Geometry check sheet. Reference: the model listing, model coordinates, mm. Face numbers are marked on the shaded views. Give positions to 0.01 mm unless a question says otherwise; leave off trailing zeros. Order: outer loops, then holes, each group sorted by start corner. A loop starts at its lowest first (then second) coordinate and runs counter-clockwise, first axis right, second up.
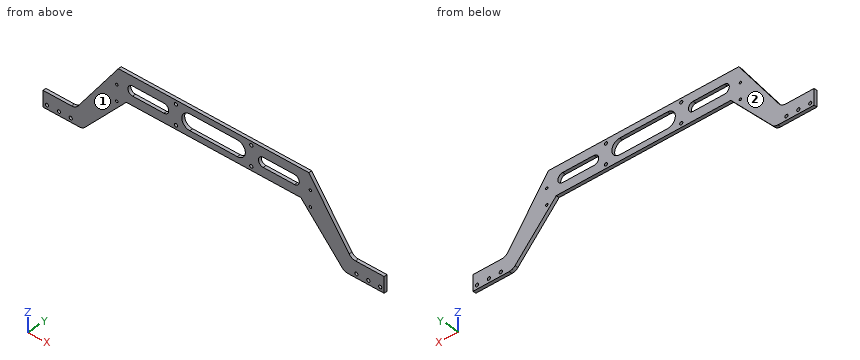
from build123d import *

# Parameters (mm, degrees)
SKETCH_2_R          = 2
EXTRUDE_1_DEPTH     = 4
SKETCH_3_R          = 1.5
CUT_EXTRUDE_1_DEPTH = 10
FILLET_1_R          = 10
CUT_EXTRUDE_2_DEPTH = 278.528827332


with BuildPart() as part:
    # 草图2 → 凸台-拉伸1 (new body)
    with BuildSketch(Plane(origin=(0, 0, 0), x_dir=(1, 0, 0), z_dir=(0, 1, 0))):
        Polygon((-72.5, -5), (167.5, -5), (221.298034327, 70), (262.5, 70), (262.5, 90), (212.5, 90), (157.5, 30), (-62.5, 30), (-117.5, 90), (-167.5, 90), (-167.5, 70), (-126.298034327, 70), align=None)
        with Locations(Location((0, 0, 0), (0, 0, 270))):
            Circle(SKETCH_2_R, mode=Mode.SUBTRACT)
        with Locations(Location((95, 0, 0), (0, 0, 270))):
            Circle(SKETCH_2_R, mode=Mode.SUBTRACT)
        with Locations(Location((95, 25, 0), (0, 0, 270))):
            Circle(SKETCH_2_R, mode=Mode.SUBTRACT)
        with Locations(Location((0, 25, 0), (0, 0, 270))):
            Circle(SKETCH_2_R, mode=Mode.SUBTRACT)
        with Locations(Location((-162.5, 85, 0), (0, 0, 270))):
            Circle(SKETCH_2_R, mode=Mode.SUBTRACT)
        with Locations(Location((-147.5, 85, 0), (0, 0, 270))):
            Circle(SKETCH_2_R, mode=Mode.SUBTRACT)
        with Locations(Location((-132.5, 85, 0), (0, 0, 270))):
            Circle(SKETCH_2_R, mode=Mode.SUBTRACT)
        with Locations(Location((227.5, 85, 0), (0, 0, 90))):
            Circle(SKETCH_2_R, mode=Mode.SUBTRACT)
        with Locations(Location((242.5, 85, 0), (0, 0, 90))):
            Circle(SKETCH_2_R, mode=Mode.SUBTRACT)
        with Locations(Location((257.5, 85, 0), (0, 0, 90))):
            Circle(SKETCH_2_R, mode=Mode.SUBTRACT)
        with BuildLine():
            Line((77.5, 2.5), (17.5, 2.5))
            ThreePointArc((17.5, 2.5), (7.5, 12.5), (17.5, 22.5))
            Line((17.5, 22.5), (77.5, 22.5))
            ThreePointArc((77.5, 22.5), (87.5, 12.5), (77.5, 2.5))
        make_face(mode=Mode.SUBTRACT)
    extrude(amount=EXTRUDE_1_DEPTH)

    # 草图3 → 切除-拉伸1 (cut)
    with BuildSketch(Plane.XZ):
        with Locations(Location((169.5, -35, 0), (0, 0, 270))):
            Circle(SKETCH_3_R)
        with Locations(Location((169.5, -15, 0), (0, 0, 270))):
            Circle(SKETCH_3_R)
        with Locations(Location((-74.5, -15, 0), (0, 0, 270))):
            Circle(SKETCH_3_R)
        with Locations(Location((-74.5, -35, 0), (0, 0, 270))):
            Circle(SKETCH_3_R)
    extrude(amount=-CUT_EXTRUDE_1_DEPTH, mode=Mode.SUBTRACT)

    # 圆角1
    fillet_1_edges = [part.edges().sort_by_distance(p)[0] for p in [
        (212.5, 2, -90),
        (221.298034327, 2, -70),
        (-126.298034327, 2, -70),
        (-117.5, 2, -90),
    ]]
    fillet(fillet_1_edges, radius=FILLET_1_R)

    # 草图4 → 切除-拉伸2 (cut, through all)
    with BuildSketch(Plane(origin=(0, 4, 0), x_dir=(1, 0, 0), z_dir=(0, 1, 0))):
        with BuildLine():
            Line((-54.5, 18.5), (-15, 18.5))
            ThreePointArc((-15, 18.5), (-9, 12.5), (-15, 6.5))
            Line((-15, 6.5), (-54.5, 6.5))
            ThreePointArc((-54.5, 6.5), (-60.5, 12.5), (-54.5, 18.5))
        make_face()
        with BuildLine():
            Line((149.5, 18.5), (110, 18.5))
            ThreePointArc((110, 18.5), (104, 12.5), (110, 6.5))
            Line((110, 6.5), (149.5, 6.5))
            ThreePointArc((149.5, 6.5), (155.5, 12.5), (149.5, 18.5))
        make_face()
    extrude(amount=-CUT_EXTRUDE_2_DEPTH, mode=Mode.SUBTRACT)


solid = part.part
Item 1: Draft check along Y on the marked faces 1 and 2. Enter one of: released by +Y, released by -Y, zero draft, split by the parting line, or undercut.
Reported:
face 1: released by -Y
face 2: released by +Y
Item 2: Gauge pin test, flat ends, axial feed: pin 1 (2 mm diameter, centred on x = 137, y = 3, fed in from -Z); pin 2 (6.5 mm diameter, centred on x = 95, z = -25, fed in from +Y). Record the tip position at first contact, or that the pin passes through.
Reported:
pin 1: stops at z = -30
pin 2: stops at y = 4
Item 3: Sectioned sample at B-B (x = 134.5). Enter the section's corners in (y, z).
Reported:
outline: (0, -30) - (4, -30) - (4, -18.5) - (0, -18.5) - close; (0, -6.5) - (4, -6.5) - (4, 5) - (0, 5) - close
Item 4: Sectioned sample at C-C (y = 2.45). Give the number of separate pieces and of enclosed holes in the cut face, and give its area (3 significant figures).
Reported:
separate pieces: 1
enclosed holes: 17
area: 11,300 mm2
Item 5: Sectioned sample at D-D (x = 200). Enter the section's corners in (y, z), and give its area (3 significant figures).
Reported:
outline: (0, -76.36) - (4, -76.36) - (4, -40.31) - (0, -40.31) - close
area: 144 mm2
Item 6: Sectioned sample at A-A (x = 54). Enter the section's corners in (y, z), and give its area (3 significant figures).
Reported:
outline: (0, -30) - (4, -30) - (4, -22.5) - (0, -22.5) - close; (0, -2.5) - (4, -2.5) - (4, 5) - (0, 5) - close
area: 60.0 mm2
Item 7: Scan lines: L1, parallel to X at y = 2.6, z = 0; L2, parallel to Z at x = -132.5, y = 2.65; L3, parallel to X at y = 1.6, z = -16. Record each from-to range of solid material in increasing order.
Reported:
L1: x = -76.09 to -2, 2 to 93, 97 to 171.09
L2: z = -90 to -87, -83 to -70
L3: x = -87.56 to -75.62, -73.38 to -59.37, -10.13 to 8.13, 86.87 to 105.13, 154.37 to 168.38, 170.62 to 182.56
